For this review, use the dimensioned drawing (mm, ordinates from the lowest corner) and the shaded views. A direction names the side the tool comes from. Coordinates: 2 decimals unless noted, no trailing zeros. Write each loop counter-clockwise with the first axis right and the second up, starting at its lowest first coordinate (ties: lowest second). Pieces come first, ordered by that corner, then holes. Notation, with made-up numbers: (-29, 79) - (9, 79) arc R27 cw to (9, 96) - close; hole circle Ø11 at (-5.75, 40). An arc over 180 degrees is marked (long way). Answer as a JSON object with one key per item and string values.
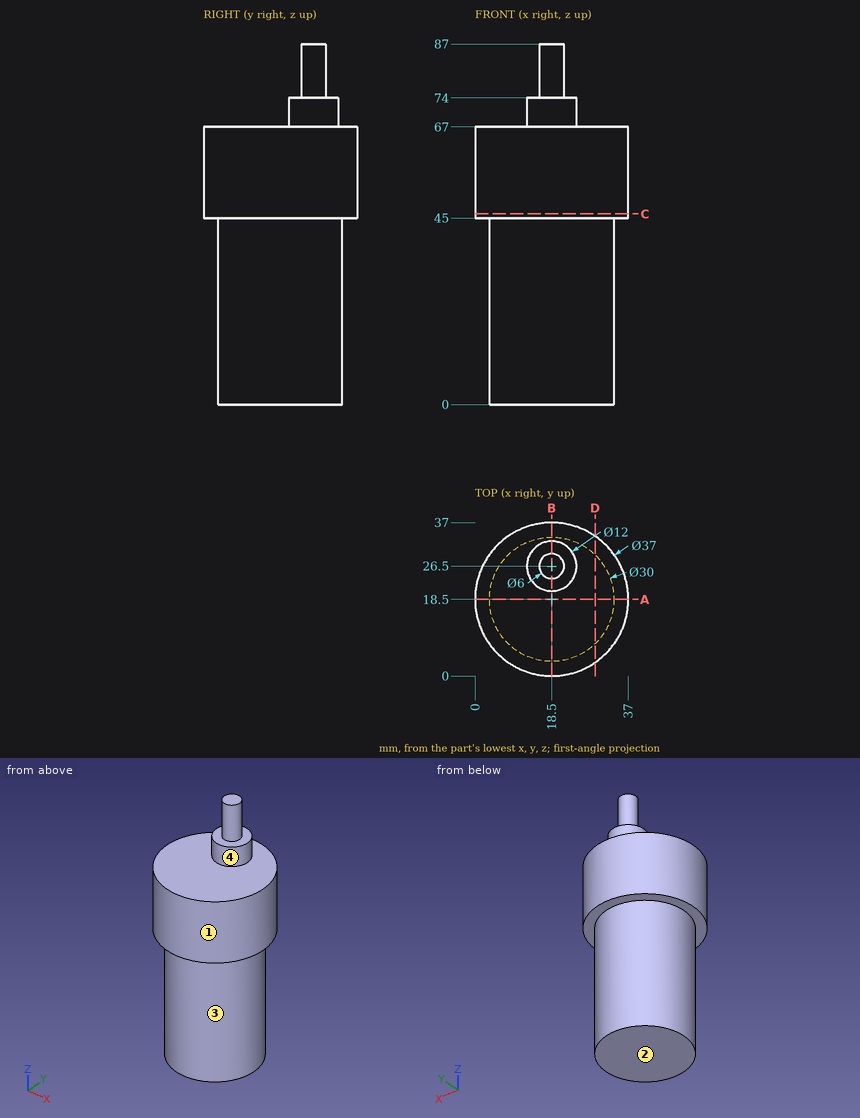
(1) For pin 1 (12 mm diameter, centred on x = 31, y = 24.5, fed in from +Z); pin 2 (2 mm diameter, centred on x = 18, z = 58, fed in from -Y); pin 3 (5 mm diameter, centred on x = 10.5, z = 15.5, fed in from -Y); pin 4 (8 mm diameter, centred on x = 21.5, y = 16.5, fed in from -Z), all flat-tipped, find the tip position at first contact; note any pin that passes through.
Solved:
{"pin 1": "stops at z = 67", "pin 2": "stops at y = 0", "pin 3": "stops at y = 4.54", "pin 4": "stops at z = 0"}
(2) Take a section at A-A, the plane y = 18.5. Write out the cut boundary in (x, z), and give its area (3 significant figures).
Solved:
{"outline": "(0, 45) - (3.5, 45) - (3.5, 0) - (33.5, 0) - (33.5, 45) - (37, 45) - (37, 67) - (0, 67) - close", "area": "2,160 mm^2"}
(3) Take a section at C-C, the plane z = 46. Write out the cut boundary in (x, y), and give its area (3 significant figures).
Solved:
{"outline": "circle Ø37 at (18.5, 18.5)", "area": "1,080 mm^2"}
(4) Take a section at D-D, the plane x = 29. Write out the cut boundary in (y, z), and give its area (3 significant figures).
Solved:
{"outline": "(3.27, 45) - (7.79, 45) - (7.79, 0) - (29.21, 0) - (29.21, 45) - (33.73, 45) - (33.73, 67) - (3.27, 67) - close", "area": "1,630 mm^2"}
(5) The part is to be moulded in two halves that separate along X. For the marked faces 1 and 2, say which applies: pulls with the +X half, pulls with the -X half, needs draft (parallel to the pull), parting line crosses it, or undercut.
Solved:
{"face 1": "parting line crosses it", "face 2": "needs draft"}
(6) To check wall thickness, follow line 1 (Z direction, x = 4, y = 12); line 2 (Z direction, x = 7, y = 16); line 3 (X direction, y = 18, z = 30). State the ranges of each line that lie inside material, in increasing order. Write a range as from..to.
Solved:
{"line 1": "z = 45..67", "line 2": "z = 0..67", "line 3": "x = 3.51..33.49"}
(7) Tool access review of the marked faces 3 and 4: name each direction out of +Z, -Z, +X, -X, +Y, -Y from which nothing blocks a thin tool from reaching the whole face with its end or side.
Solved:
{"face 3": "-Z", "face 4": "+Z"}
(8) Take a section at B-B, the plane x = 18.5. Write out the cut boundary in (y, z), and give its area (3 significant figures).
Solved:
{"outline": "(0, 45) - (3.5, 45) - (3.5, 0) - (33.5, 0) - (33.5, 45) - (37, 45) - (37, 67) - (32.5, 67) - (32.5, 74) - (29.5, 74) - (29.5, 87) - (23.5, 87) - (23.5, 74) - (20.5, 74) - (20.5, 67) - (0, 67) - close", "area": "2,330 mm^2"}
